```python
from build123d import *

# Parameters (mm, degrees)
SKETCH1_W           = 24
SKETCH1_H           = 24
BOSS_EXTRUDE1_DEPTH = 250
SKETCH2_W           = 3.6
SKETCH2_H           = 12
CUT_EXTRUDE1_DEPTH  = 250
SKETCH8_W           = 8.4
SKETCH8_H           = 18
BOSS_EXTRUDE2_DEPTH = 18
SKETCH6_R           = 2.1
SKETCH6_R_2         = 4.5
CUT_EXTRUDE3_DEPTH  = 8.4


with BuildPart() as part:
    # Sketch1 → Boss-Extrude1 (new body)
    with BuildSketch(Plane.XY):
        Rectangle(SKETCH1_W, SKETCH1_H)
    extrude(amount=BOSS_EXTRUDE1_DEPTH)

    # Sketch2 → Cut-Extrude1 (cut)
    with BuildSketch(Plane.XY.offset(250)):
        with Locations((1.8, 6)):
            Rectangle(SKETCH2_W, SKETCH2_H)
    cut_extrude1 = extrude(amount=-CUT_EXTRUDE1_DEPTH, mode=Mode.SUBTRACT)

    # Mirror1: Cut-Extrude1 across plane
    add(cut_extrude1.mirror(Plane(origin=(0, 0, 0), x_dir=(0, 0, 1), z_dir=(1, 0, 0))), mode=Mode.SUBTRACT)

    # Sketch8 → Boss-Extrude2 (add)
    with BuildSketch(Plane(origin=(0, 12, 0), x_dir=(1, 0, 0), z_dir=(0, 1, 0))):
        with Locations((7.8, -9)):
            Rectangle(SKETCH8_W, SKETCH8_H)
    extrude(amount=BOSS_EXTRUDE2_DEPTH)

    # Sketch6 → Cut-Extrude3 (cut)
    with BuildSketch(Plane(origin=(12, 0, 0), x_dir=(0, 0, -1), z_dir=(1, 0, 0))):
        with Locations(Location((-3.5, -8.5, 0), (0, 0, 90))):
            Circle(SKETCH6_R)
        with Locations(Location((-16.149110641, 6, 0), (0, 0, 90))):
            Circle(SKETCH6_R_2)
        with Locations(Location((-13.459703626, 25.053007372, 0), (0, 0, 90))):
            Circle(SKETCH6_R)
    extrude(amount=-CUT_EXTRUDE3_DEPTH, mode=Mode.SUBTRACT)


solid = part.part
```
Geometry: final body of the model. Coordinates: model frame, mm. A direction names the side the tool comes from. Round coordinates to 2 decimals unless told otherwise and drop trailing zeros. Order: outer loops, then holes, each group sorted by start corner. A loop starts at its lowest first (then second) coordinate and runs counter-clockwise, first axis right, second up. Notation, with made-up numbers: (-21, -0.5) -> (8, -0.5) arc R28 ccw to (8, 22.5) -> close; hole circle Ø7 at (-3, 84). An arc over 180 degrees is marked (long way). Use one line per item in the form item = value. Start each with the question number.
1. Cut plane B-B (z = 118). Return the cut outline in (x, y).
2. Draft query along Y for faces 1 (the face through (7.859, 5.024, 11.756)), 2 (the face through (8, 12, 132)), 3 (the face through (-3.6, 6, 127)). Return one class per face: pulls with the +Y half, pulls with the -Y half, needs draft (parallel to the pull), parting line crosses it, or undercut.
3. Cut plane D-D (x = -9.75). Return the cut outline in (y, z).
4. Cut plane A-A (y = 6). Return the cut outline in (x, z), then the cut area to 3 significant figures.
5. Pin query (flat end, axial travel): pin 1 Ø2.5 at (x, z) = (-7.5, 79.5) entering from +Y; pin 2 Ø4.5 at (y, z) = (-8.5, 3.5) entering from +X; pin 3 Ø2.5 at (x, y) = (8.5, 17) entering from +Z; pin 4 Ø1.5 at (x, z) = (1.5, 112.5) entering from +Y. Return the tip coordinate at first contact, or that it passes through.
6. Cut plane C-C (y = 25). Return the cut outline in (x, z).
7. Line query: probe 1 along Z at (x, y) = (9, 6); probe 2 along X at (y, z) = (7.5, 132.5); probe 3 along Z at (x, y) = (9.25, -8.5). Output: solid intervals per line, ascending.
8. Reachability of faces 4 (the face through (7.859, -10.166, 2.222)), 5 (the face through (8, 21, 18)), 6 (the face through (0, 0, 127)), 7 (the face through (8, 30, 9)) from +Z, -Z, +X, -X, +Y, -Y: full face, straight path, thin tool, end or side. Return the list, or none.
Solution:
q1.outline = (-12, -12) -> (12, -12) -> (12, 12) -> (3.6, 12) -> (3.6, 0) -> (-3.6, 0) -> (-3.6, 12) -> (-12, 12) -> close
q2.face_1 = undercut
q2.face_2 = pulls with the +Y half
q2.face_3 = needs draft
q3.outline = (-12, 0) -> (12, 0) -> (12, 250) -> (-12, 250) -> close
q4.outline = (-12, 0) -> (-3.6, 0) -> (-3.6, 250) -> (-12, 250) -> close; (3.6, 0) -> (12, 0) -> (12, 11.65) -> (3.6, 11.65) -> close; (3.6, 20.65) -> (12, 20.65) -> (12, 250) -> (3.6, 250) -> close
q4.area = 4,120 mm^2
q5.pin_1 = 12
q5.pin_2 = 12
q5.pin_3 = 18
q5.pin_4 = 0
q6.outline = (3.6, 0) -> (12, 0) -> (12, 11.36) -> (3.6, 11.36) -> close; (3.6, 15.56) -> (12, 15.56) -> (12, 18) -> (3.6, 18) -> close
q7.probe_1 = 0 to 11.65, 20.65 to 250
q7.probe_2 = -12 to -3.6, 3.6 to 12
q7.probe_3 = 0 to 1.4, 5.6 to 250
q8.face_4 = +X
q8.face_5 = +Z, +X, -X, +Y
q8.face_6 = +Z, -Z, +Y
q8.face_7 = +Z, -Z, +X, -X, +Y
